from build123d import *

# Parameters (mm, degrees)
F0_R     = 95
F0_R_2   = 6.6
F0_R_3   = 2.5
F0_R_4   = 45
F1_DEPTH = 5


with BuildPart() as f1:
    # F0 (on Top) → F1 (new body)
    with BuildSketch(Plane.XY):
        Circle(F0_R)
        with Locations((-64.671567, -26.78784)):
            Circle(F0_R_2, mode=Mode.SUBTRACT)
        with Locations((-36, -36)):
            Circle(F0_R_3, mode=Mode.SUBTRACT)
        with Locations((0, -50)):
            Circle(F0_R_3, mode=Mode.SUBTRACT)
        with Locations((36, -36)):
            Circle(F0_R_3, mode=Mode.SUBTRACT)
        with Locations((64.671567, -26.78784)):
            Circle(F0_R_2, mode=Mode.SUBTRACT)
        with Locations((-50, 0)):
            Circle(F0_R_3, mode=Mode.SUBTRACT)
        with Locations((-36, 36)):
            Circle(F0_R_3, mode=Mode.SUBTRACT)
        with Locations((-42.6133, 55.534734)):
            Circle(F0_R_2, mode=Mode.SUBTRACT)
        Circle(F0_R_4, mode=Mode.SUBTRACT)
        with Locations((36, 36)):
            Circle(F0_R_3, mode=Mode.SUBTRACT)
        with Locations((50, 0)):
            Circle(F0_R_3, mode=Mode.SUBTRACT)
        with Locations((0, 50)):
            Circle(F0_R_3, mode=Mode.SUBTRACT)
        with Locations((42.6133, 55.534734)):
            Circle(F0_R_2, mode=Mode.SUBTRACT)
    extrude(amount=F1_DEPTH)


solid = f1.part
For this review, take the finished solid that the model builds, in its own axes (mm). Coordinates: 2 decimals unless noted, no trailing zeros. Order: outer loops, then holes, each group sorted by start corner. A loop starts at its lowest first (then second) coordinate and runs counter-clockwise, first axis right, second up. Notation, with made-up numbers: (81, 5) - (117, 5) arc R12 ccw to (117, 26) - close; hole circle Ø5 at (14.25, 36). An arc over 180 degrees is marked (long way). Use one line per item in the form item = value.
Q1. Consider section B-B (y = 24.5). Give the boundary of the cut face in (x, z).
Checked values:
outline = (-91.79, 0) - (-37.75, 0) - (-37.75, 5) - (-91.79, 5) - close; (37.75, 0) - (91.79, 0) - (91.79, 5) - (37.75, 5) - close
Q2. Consider section C-C (z = 1.8). Give the number of separate pieces and of enclosed holes in the cut face, then the cut area to 3 significant figures.
Checked values:
separate_pieces = 1
enclosed_holes = 13
area = 21,300 mm2
Q3. For probe 1 along Y at (x, z) = (-1, 3.75); probe 2 along Y at (x, z) = (-48.5, 1.7); probe 3 along X at (y, z) = (-29, 1.25), list the stretches that pass through material, from the lowest coordinate up. Write a range as from..to.
Checked values:
probe_1 = -94.99..-52.29, -47.71..-44.99, 44.99..47.71, 52.29..94.99
probe_2 = -81.69..-2, 2..52.55, 58.52..81.69
probe_3 = -90.47..-70.89, -58.45..-34.41, 34.41..58.45, 70.89..90.47
Q4. Consider section D-D (y = -24). Give the boundary of the cut face in (x, z).
Checked values:
outline = (-91.92, 0) - (-70.65, 0) - (-70.65, 5) - (-91.92, 5) - close; (-58.69, 0) - (-38.07, 0) - (-38.07, 5) - (-58.69, 5) - close; (38.07, 0) - (58.69, 0) - (58.69, 5) - (38.07, 5) - close; (70.65, 0) - (91.92, 0) - (91.92, 5) - (70.65, 5) - close
Q5. For P1, Ø3, axis at x = 36, y = 36, coming from the +Z side; P2, Ø2, axis at y = 64.5, z = 4, coming from the +X side; P3, Ø2, axis at y = -60.5, z = 1.5, coming from the -X side; P4, Ø1.5, axis at y = 71, z = 3.5, coming from the +X side, all flat-tipped, find the tip position at first contact; note any pin that passes through.
Checked values:
P1 = through
P2 = 70.66
P3 = -74.06
P4 = 63.95
Q6. Draft analysis for pull direction X (two halves, no side actions). For faces 1 (the flat face through (41, -20, 5)), 2 (the cylindrical face through (70.768, -29.316, 2.465)), 3 (the cylindrical face through (-20.59, -92.74, 2.46)), state which applies: +X half, -X half, draft (parallel to the pull), parting line (faces both ways), or undercut.
Checked values:
face_1 = draft
face_2 = undercut
face_3 = parting line
Q7. Consider section A-A (x = 0). Give the boundary of the cut face in (y, z), then the cut area to 3 significant figures.
Checked values:
outline = (-95, 0) - (-52.5, 0) - (-52.5, 5) - (-95, 5) - close; (-47.5, 0) - (-45, 0) - (-45, 5) - (-47.5, 5) - close; (45, 0) - (47.5, 0) - (47.5, 5) - (45, 5) - close; (52.5, 0) - (95, 0) - (95, 5) - (52.5, 5) - close
area = 450 mm2
